Check sheet for the modelled part. Datum: model origin and axes. Units: mm. A direction names the side the tool comes from. Give positions to 0.01 mm unless a question says otherwise; leave off trailing zeros. Write each loop counter-clockwise with the first axis right and the second up, starting at its lowest first coordinate (ties: lowest second). Pieces come first, ordered by that corner, then holes. Notation, with made-up numbers: (-14, -10.75) -> (12, -10.75) arc R32 cw to (12, 15.25) -> close; hole circle Ø1 at (53.5, 2). An arc over 180 degrees is marked (long way). Answer as a JSON object with one key per item and string values.
from build123d import *

# Parameters (mm, degrees)
SKETCH2_R           = 37.5
SKETCH2_R_2         = 5.35
BOSS_EXTRUDE2_DEPTH = 8
SKETCH14_R          = 2
CUT_EXTRUDE6_DEPTH  = 54.633012222
SKETCH3_R           = 20.71
CUT_EXTRUDE2_DEPTH  = 6.5
SKETCH7_R           = 12.5
SKETCH7_R_2         = 10.5
BOSS_EXTRUDE4_DEPTH = 50.8
SKETCH10_R          = 12.5
BOSS_EXTRUDE5_DEPTH = 2.01
BOSS_EXTRUDE5_DRAFT = -75
SKETCH11_R          = 10.5
CUT_EXTRUDE3_DEPTH  = 81.686777727
BOSS_EXTRUDE6_START = 3
SKETCH12_R          = 20.001422123
SKETCH12_R_2        = 10.5
BOSS_EXTRUDE6_DEPTH = 3
SKETCH13_R          = 13.1
CUT_EXTRUDE4_DEPTH  = 2.5
SKETCH17_R          = 4.5
CUT_EXTRUDE8_DEPTH  = 3.75
SKETCH18_R          = 37.5
CUT_EXTRUDE9_DEPTH  = 2
SKETCH19_R          = 27.5
CUT_EXTRUDE10_DEPTH = 3
CUT_EXTRUDE11_DEPTH = 3


with BuildPart() as part:
    # Sketch2 → Boss-Extrude2 (new body)
    with BuildSketch(Plane.XY):
        Circle(SKETCH2_R)
        Circle(SKETCH2_R_2, mode=Mode.SUBTRACT)
    extrude(amount=BOSS_EXTRUDE2_DEPTH)

    # Sketch14 → Cut-Extrude6 (cut, through all)
    with BuildSketch(Plane.XY):
        with Locations((0, 33.75)):
            Circle(SKETCH14_R)
        with Locations((-23.864853865, 23.864853865)):
            Circle(SKETCH14_R)
        with Locations((-33.75, 0)):
            Circle(SKETCH14_R)
        with Locations((-23.864853865, -23.864853865)):
            Circle(SKETCH14_R)
        with Locations((0, -33.75)):
            Circle(SKETCH14_R)
        with Locations((23.864853865, -23.864853865)):
            Circle(SKETCH14_R)
        with Locations((33.75, 0)):
            Circle(SKETCH14_R)
        with Locations((23.864853865, 23.864853865)):
            Circle(SKETCH14_R)
    extrude(amount=CUT_EXTRUDE6_DEPTH, mode=Mode.SUBTRACT)

    # Sketch3 → Cut-Extrude2 (cut)
    with BuildSketch(Plane.XY):
        with Locations(Location((0, 0, 0), (0, 0, 180))):
            Circle(SKETCH3_R)
    extrude(amount=CUT_EXTRUDE2_DEPTH, mode=Mode.SUBTRACT)

    # Sketch7 → Boss-Extrude4 (add)
    with BuildSketch(Plane.XY.offset(8)):
        Circle(SKETCH7_R)
        Circle(SKETCH7_R_2, mode=Mode.SUBTRACT)
    extrude(amount=BOSS_EXTRUDE4_DEPTH)


with BuildPart() as boss_extrude5_tool:
    # Sketch10 → Boss-Extrude5 (with draft: the straight prism first)
    with BuildSketch(Plane.XY.offset(58.8)):
        Circle(SKETCH10_R)
    extrude(amount=BOSS_EXTRUDE5_DEPTH)
    # Boss-Extrude5: the draft: its side faces are tilted about the plane it starts from
    boss_extrude5_sides = [boss_extrude5_tool.faces().sort_by_distance(p)[0] for p in [
        (-12.5, 0, 59.805),
    ]]
    draft(boss_extrude5_sides, Plane.XY.offset(58.8), BOSS_EXTRUDE5_DRAFT)


with BuildPart() as part_1:
    add(part.part)

    # Boss-Extrude5: add boss_extrude5_tool
    add(boss_extrude5_tool.part)

    # Sketch11 → Cut-Extrude3 (cut, through all)
    with BuildSketch(Plane.XY.offset(60.81)):
        Circle(SKETCH11_R)
    extrude(amount=-CUT_EXTRUDE3_DEPTH, mode=Mode.SUBTRACT)

    # Sketch12 → Boss-Extrude6 (add)
    with BuildSketch(Plane.XY.offset(60.81).offset(BOSS_EXTRUDE6_START)):
        Circle(SKETCH12_R)
        Circle(SKETCH12_R_2, mode=Mode.SUBTRACT)
    extrude(amount=-BOSS_EXTRUDE6_DEPTH)

    # Sketch13 → Cut-Extrude4 (cut)
    with BuildSketch(Plane.XY.offset(63.81)):
        Circle(SKETCH13_R)
    extrude(amount=-CUT_EXTRUDE4_DEPTH, mode=Mode.SUBTRACT)

    # Sketch17 → Cut-Extrude8 (cut)
    with BuildSketch(Plane.XY.offset(8)):
        with Locations((-23.864853865, 23.864853865)):
            Circle(SKETCH17_R)
        with Locations((-33.75, 0)):
            Circle(SKETCH17_R)
        with Locations((0, 33.75)):
            Circle(SKETCH17_R)
        with Locations((23.864853865, 23.864853865)):
            Circle(SKETCH17_R)
        with Locations((33.75, 0)):
            Circle(SKETCH17_R)
        with Locations((23.864853865, -23.864853865)):
            Circle(SKETCH17_R)
        with Locations((0, -33.75)):
            Circle(SKETCH17_R)
        with Locations((-23.864853865, -23.864853865)):
            Circle(SKETCH17_R)
    extrude(amount=-CUT_EXTRUDE8_DEPTH, mode=Mode.SUBTRACT)

    # Sketch18 → Cut-Extrude9 (cut)
    with BuildSketch(Plane(origin=(0, 0, 0), x_dir=(-1, 0, 0), z_dir=(0, 0, -1))):
        Circle(SKETCH18_R)
    extrude(amount=-CUT_EXTRUDE9_DEPTH, mode=Mode.SUBTRACT)

    # Sketch19 → Cut-Extrude10 (cut)
    with BuildSketch(Plane(origin=(0, 0, 2), x_dir=(-1, 0, 0), z_dir=(0, 0, -1))):
        Circle(SKETCH19_R)
    extrude(amount=-CUT_EXTRUDE10_DEPTH, mode=Mode.SUBTRACT)

    # Sketch21 → Cut-Extrude11 (cut)
    with BuildSketch(Plane(origin=(0, 0, 2), x_dir=(-1, 0, 0), z_dir=(0, 0, -1))):
        with BuildLine():
            ThreePointArc((-19.445436483, -19.445436483), (-25.406687144, -10.52379439), (-27.5, 0))
            Line((-27.5, 0), (-35.190042838, -4.680906432))
            ThreePointArc((-35.190042838, -4.680906432), (-32.79655916, -13.588072242), (-28.189320962, -21.578048653))
            Line((-28.189320962, -21.578048653), (-19.445436483, -19.445436483))
        make_face()
        with BuildLine():
            Line((-35.190844537, 4.674875482), (-27.5, 0))
            ThreePointArc((-27.5, 0), (-25.406687144, 10.52379439), (-19.445436483, 19.445436483))
            Line((-19.445436483, 19.445436483), (-28.193018602, 21.573217241))
            ThreePointArc((-28.193018602, 21.573217241), (-32.798887407, 13.582451357), (-35.190844537, 4.674875482))
        make_face()
        with BuildLine():
            Line((-21.578048653, 28.189320962), (-19.445436483, 19.445436483))
            ThreePointArc((-19.445436483, 19.445436483), (-10.52379439, 25.406687144), (0, 27.5))
            Line((0, 27.5), (-4.680906432, 35.190042838))
            ThreePointArc((-4.680906432, 35.190042838), (-13.588072242, 32.79655916), (-21.578048653, 28.189320962))
        make_face()
        with BuildLine():
            Line((4.674875482, 35.190844537), (0, 27.5))
            ThreePointArc((0, 27.5), (10.52379439, 25.406687144), (19.445436483, 19.445436483))
            Line((19.445436483, 19.445436483), (21.573217241, 28.193018602))
            ThreePointArc((21.573217241, 28.193018602), (13.582451357, 32.798887407), (4.674875482, 35.190844537))
        make_face()
        with BuildLine():
            Line((28.189320962, 21.578048653), (19.445436483, 19.445436483))
            ThreePointArc((19.445436483, 19.445436483), (25.406687144, 10.52379439), (27.5, 0))
            Line((27.5, 0), (35.190042838, 4.680906432))
            ThreePointArc((35.190042838, 4.680906432), (32.79655916, 13.588072242), (28.189320962, 21.578048653))
        make_face()
        with BuildLine():
            ThreePointArc((27.5, 0), (25.406687144, -10.52379439), (19.445436483, -19.445436483))
            Line((19.445436483, -19.445436483), (28.193018602, -21.573217241))
            ThreePointArc((28.193018602, -21.573217241), (32.798887407, -13.582451357), (35.190844537, -4.674875482))
            Line((35.190844537, -4.674875482), (27.5, 0))
        make_face()
        with BuildLine():
            ThreePointArc((19.445436483, -19.445436483), (10.52379439, -25.406687144), (0, -27.5))
            Line((0, -27.5), (4.680906432, -35.190042838))
            ThreePointArc((4.680906432, -35.190042838), (13.588072242, -32.79655916), (21.578048653, -28.189320962))
            Line((21.578048653, -28.189320962), (19.445436483, -19.445436483))
        make_face()
        with BuildLine():
            ThreePointArc((0, -27.5), (-10.52379439, -25.406687144), (-19.445436483, -19.445436483))
            Line((-19.445436483, -19.445436483), (-21.573217241, -28.193018602))
            ThreePointArc((-21.573217241, -28.193018602), (-13.582451357, -32.798887407), (-4.674875482, -35.190844537))
            Line((-4.674875482, -35.190844537), (0, -27.5))
        make_face()
    extrude(amount=-CUT_EXTRUDE11_DEPTH, mode=Mode.SUBTRACT)


solid = part_1.part
1. Sectioned sample at A-A, the plane z = 44. Enter the section's corners in (x, y), plus the area to 3 significant figures.
Determined:
{"outline": "circle Ø25 at (0, 0); hole circle Ø21 at (0, 0)", "area": "145 mm^2"}
2. Access from +Z, -Z, +X, -X, +Y, -Y to the whole of each face (thin tool, end or side, straight path). Record for faces 4 (the face through (-1.705, 12.989, 62.578)), 5 (the face through (10, 3.2, 34.3)), 6 (the face through (-32.846, 13.468, 3.479)).
Determined:
{"face 4": "+Z", "face 5": "+Z, -Z", "face 6": "-Z"}
3. Scan lines: L1, parallel to Y at x = 0, z = 7; L2, parallel to Y at x = -0.5, z = 21.5; L3, parallel to Z at x = 1, y = -14.5. Record each from-to range of solid material in increasing order. Write a range as [from, to].
Determined:
{"L1": "[-29.25, -10.5], [10.5, 29.25]", "L2": "[-12.49, -10.49], [10.49, 12.49]", "L3": "[6.5, 8], [59.35, 63.81]"}
4. Go/stop test with flat-tipped pins: P1, Ø6.5, axis at x = 23, y = -22.5, coming from the +Z side; P2, Ø4, axis at x = 25.5, y = 24.5, coming from the +Z side; P3, Ø8, axis at x = -21.5, y = 3.5, coming from the +Z side; P4, Ø8, axis at y = -13, z = 51.5, coming from the -X side. Record where each tip stops, or that it passes through.
Determined:
{"P1": "z = 8", "P2": "z = 4.25", "P3": "z = 63.81", "P4": "x = -8.67"}
5. Mould release check, pull along Z, two halves, no side actions. Record for faces 1 (the face through (-13.7, 32.75, 3.48)), 2 (the face through (0, 28, 2)), 3 (the face through (16, 1, 8)): released by +Z, released by -Z, zero draft, split by the parting line, or undercut.
Determined:
{"face 1": "zero draft", "face 2": "released by -Z", "face 3": "undercut"}
